Read the model definition and answer for the solid it produces. Units are mm, in the model's axes. A direction names the side the tool comes from. Round coordinates to 2 decimals unless told otherwise and drop trailing zeros. Write each loop counter-clockwise with the first axis right and the second up, starting at its lowest first coordinate (ties: lowest second). Pieces come first, ordered by that corner, then holes. Notation, with made-up numbers: (-19.5, -35) -> (27.5, -35) arc R15 ccw to (27.5, -14) -> close; hole circle Ø10 at (77, 68). An arc over 180 degrees is marked (long way). Return JSON: item names as keys, results as strings.
from build123d import *

# Parameters (mm, degrees)
ESQUISSE1_W             = 204.52
ESQUISSE1_H             = 166.42
BOSS_EXTRU_1_DEPTH      = 10
CHANFREIN1_SIZE         = 15
ENL_V_MAT_EXTRU_1_DEPTH = 2
ENL_V_MAT_EXTRU_2_DEPTH = 4
ESQUISSE4_R             = 1.65
ENL_V_MAT_EXTRU_3_DEPTH = 9
ESQUISSE5_R             = 3.8
ENL_V_MAT_EXTRU_4_DEPTH = 2.8
ESQUISSE6_W             = 16.1
ESQUISSE6_H             = 3
BOSS_EXTRU_2_DEPTH      = 2


with BuildPart() as part:
    # Esquisse1 → Boss.-Extru.1 (new body)
    with BuildSketch(Plane.XY):
        Rectangle(ESQUISSE1_W, ESQUISSE1_H)
    extrude(amount=BOSS_EXTRU_1_DEPTH)

    # Chanfrein1
    chanfrein1_edges = [part.edges().sort_by_distance(p)[0] for p in [
        (-102.26, 83.21, 5),
        (102.26, 83.21, 5),
        (102.26, -83.21, 5),
        (-102.26, -83.21, 5),
    ]]
    chamfer(chanfrein1_edges, length=CHANFREIN1_SIZE)

    # Esquisse2 → Enlèv. mat.-Extru.1 (cut)
    with BuildSketch(Plane.XY.offset(10)):
        Polygon((86.431572875, -81.21), (100.26, -67.381572875), (100.26, 67.381572875), (86.431572875, 81.21), (-86.431572875, 81.21), (-100.26, 67.381572875), (-100.26, -67.381572875), (-86.431572875, -81.21), align=None)
    extrude(amount=-ENL_V_MAT_EXTRU_1_DEPTH, mode=Mode.SUBTRACT)

    # Esquisse3 → Enlèv. mat.-Extru.2 (cut)
    with BuildSketch(Plane.XY.offset(8)):
        Polygon((-81.611572875, 81.21), (-81.611572875, 68.762452403), (-87.812452403, 62.561572875), (-100.26, 62.561572875), (-100.26, -62.561572875), (-87.812452403, -62.561572875), (-81.611572875, -68.762452403), (-81.611572875, -81.21), (81.611572875, -81.21), (81.611572875, -68.762452403), (87.812452403, -62.561572875), (100.26, -62.561572875), (100.26, 62.561572875), (87.812452403, 62.561572875), (81.611572875, 68.762452403), (81.611572875, 81.21), align=None)
    extrude(amount=-ENL_V_MAT_EXTRU_2_DEPTH, mode=Mode.SUBTRACT)

    # Esquisse4 → Enlèv. mat.-Extru.3 (cut, through all)
    with BuildSketch(Plane.XY.offset(8)):
        with Locations((-87.06, 68.01)):
            Circle(ESQUISSE4_R)
        with Locations((-87.06, -68.01)):
            Circle(ESQUISSE4_R)
        with Locations((87.06, -68.01)):
            Circle(ESQUISSE4_R)
        with Locations((87.06, 68.01)):
            Circle(ESQUISSE4_R)
    extrude(amount=-ENL_V_MAT_EXTRU_3_DEPTH, mode=Mode.SUBTRACT)

    # Esquisse5 → Enlèv. mat.-Extru.4 (cut)
    with BuildSketch(Plane(origin=(0, 0, 0), x_dir=(-1, 0, 0), z_dir=(0, 0, -1))):
        with Locations((87.06, 68.01)):
            Circle(ESQUISSE5_R)
        with Locations((-87.06, 68.01)):
            Circle(ESQUISSE5_R)
        with Locations((-87.06, -68.01)):
            Circle(ESQUISSE5_R)
        with Locations((87.06, -68.01)):
            Circle(ESQUISSE5_R)
    extrude(amount=-ENL_V_MAT_EXTRU_4_DEPTH, mode=Mode.SUBTRACT)

    # Esquisse6 → Boss.-Extru.2 (add)
    with BuildSketch(Plane.XZ.offset(83.21)):
        with Locations((0, 8.5)):
            Rectangle(ESQUISSE6_W, ESQUISSE6_H)
    extrude(amount=BOSS_EXTRU_2_DEPTH)


solid = part.part
Item 1: Section B-B (y = 54) is taken. Give the vertices of the cut face in (x, z).
Worked answers:
{"outline": "(-102.26, 0) -> (102.26, 0) -> (102.26, 10) -> (100.26, 10) -> (100.26, 4) -> (-100.26, 4) -> (-100.26, 10) -> (-102.26, 10) -> close"}
Item 2: For a pull along X with two mould halves and no side action, classify faces 1 (the flat face through (-1, 1, 0)), 2 (the flat face through (94.865, -75.605, 4.93)), 3 (the flat face through (94, 62.562, 6)) as released by +X, released by -X, zero draft, split by the parting line, or undercut.
Worked answers:
{"face 1": "zero draft", "face 2": "released by +X", "face 3": "undercut"}
Item 3: A tool of negligible diameter and unlimited length cuts with its end or side. For faces 4 (the flat face through (-94.655, -75.815, 4.93)), 5 (the flat face through (93.44, 74.2, 9.01)), 6 (the flat face through (-89, 67, 2.8)), from which of +Z, -Z, +X, -X, +Y, -Y can it reach the whole face along a straight path? Write none if from no direction.
Worked answers:
{"face 4": "+Z, -Z, -X, -Y", "face 5": "+Z", "face 6": "-Z"}
Item 4: Flat-ended cylindrical pins translate along their axes: pin 1 (2 mm diameter, centred on x = 92.5, z = 5.5, fed in from +Y); pin 2 (2 mm diameter, centred on y = 75.5, z = 6.5, fed in from -X); pin 3 (7 mm diameter, centred on x = -87.06, y = 68.01, fed in from -Z). Find the tip coordinate at first contact, or state that the pin passes through.
Worked answers:
{"pin 1": "stops at y = 78.97", "pin 2": "stops at x = -95.97", "pin 3": "stops at z = 2.8"}
Item 5: Section A-A (x = 13.5) is taken. Give the vertices of the cut face in (y, z).
Worked answers:
{"outline": "(-83.21, 0) -> (83.21, 0) -> (83.21, 10) -> (81.21, 10) -> (81.21, 4) -> (-81.21, 4) -> (-81.21, 10) -> (-83.21, 10) -> close"}
Item 6: Straight lines are drawn through the part: L1, parallel to Y at x = -87.06, z = 0.8; L2, parallel to X at y = -10, z = 7.25; L3, parallel to Y at x = 65, z = 8. For each, find the intervals that lie inside material, in ascending order. Write a range as [from, to].
Worked answers:
{"L1": "y = [-83.21, -71.81], [-64.21, 64.21], [71.81, 83.21]", "L2": "x = [-102.26, -100.26], [100.26, 102.26]", "L3": "y = [-83.21, -81.21], [81.21, 83.21]"}
